Source: CAD feature listing. Evaluate the final solid. Frame: model axes, mm. A direction names the side the tool comes from. Round coordinates to 2 decimals unless told otherwise and drop trailing zeros. Order: outer loops, then holes, each group sorted by start corner. A loop starts at its lowest first (then second) coordinate and runs counter-clockwise, first axis right, second up. Notation, with made-up numbers: (-32, 0.25) -> (9, 0.25) arc R23 ccw to (9, 31.25) -> close; hole circle Ø3 at (-37.5, 51.25). An arc over 180 degrees is marked (long way). Answer as CSV lines item,"result". Start each with the question number.
(1) Contact query for flat-ended pins moving along their axis: P1, Ø6, axis at x = 6, z = -6, coming from the -Y side; P2, Ø2, axis at y = 19, z = 3, coming from the +X side; P3, Ø4, axis at y = 122, z = -4.5, coming from the +X side; P4, Ø8, axis at x = 8, z = -4, coming from the +Y side. Output: stop coordinate, or through.
(2) Section query A-A (y = 113). Output: boundary loops of the cut face in (x, z), plus the area to 3 significant figures.
(3) Pull-direction query (Y, two-part tool) for faces 5 (the flat face through (3, 119, 3)), 6 (the flat face through (9.93, 92.26, 0)), 7 (the cylindrical face through (-2.17, 124.39, 9.76)); classes: +Y half, -Y half, draft (parallel to the pull), parting line (faces both ways), or undercut.
(4) Line query: line 1 along Y through (x, z) = (-2, 4); line 2 along Y through (x, z) = (11, -1.5); line 3 along X through (y, z) = (82.5, -1.25). Output: solid intervals per line, ascending. Write a range as from..to.
(5) Set-up query: faces 1 (the flat face through (4, 122, 0.2)), 2 (the flat face through (2, 123.9, 2)), 3 (the flat face through (-0.2, 122, -4)), 4 (the flat face through (-0.003, 95.715, -9.877)). Return all of +Z, -Z, +X, -X, +Y, -Y with unobstructed straight access to the full face (end or side cutting, diameter ignored); none if empty.
```python
from build123d import *

# Parameters (mm, degrees)
EXTRUDE_START         = -0.2
EXTRUDE_1_OUTLINE_W   = 0.4
EXTRUDE_1_OUTLINE_H   = 3.7
EXTRUDE_1_DEPTH       = 0.4
EXTRUDE_START_2       = -7.2
EXTRUDE_1_2_OUTLINE_W = 0.4
EXTRUDE_1_2_OUTLINE_H = 3.7
EXTRUDE_1_2_DEPTH     = 7
EXTRUDE_START_3       = 119
EXTRUDE_1_3_OUTLINE_R = 14.4
EXTRUDE_1_3_DEPTH     = 1.2
EXTRUDE_1_4_OUTLINE_R = 14.5
EXTRUDE_1_4_DEPTH     = 0.85
EXTRUDE_START_4       = 123.9
EXTRUDE_1_5_OUTLINE_R = 10
EXTRUDE_1_5_DEPTH     = 1
EXTRUDE_1_6_DEPTH     = 0.4
CUT_EXTRUDE_1_DEPTH   = 129.075368436
CUT_EXTRUDE_2_DEPTH   = 129.075368436
DRAFT_1_ANGLE         = 63.434948823
DRAFT_2_ANGLE         = 63.434948823
RIB_1_REACH           = 130.053
SKETCH_4_WALL_W       = 267.026519706
SKETCH_4_WALL_H       = 0.4
RIB_2_REACH           = 130.053
SKETCH_5_WALL_W       = 267.026519706
SKETCH_5_WALL_H       = 0.4
RIB_3_REACH           = 130.053
SKETCH_6_WALL_W       = 267.026519706
SKETCH_6_WALL_H       = 0.4
RIB_4_REACH           = 130.053
SKETCH_7_WALL_W       = 261.805134662
SKETCH_7_WALL_H       = 0.4
RIB_5_REACH           = 130.053
SKETCH_8_WALL_W       = 261.805134662
SKETCH_8_WALL_H       = 0.4
RIB_6_REACH           = 130.053
SKETCH_9_WALL_W       = 261.805134662
SKETCH_9_WALL_H       = 0.4
RIB_START             = -0.2
RIB_7_DEPTH           = 0.4
RIB_8_DEPTH           = 0.4
FILLET_1_R            = 0.4
FILLET_2_R            = 2
FILLET_3_R            = 15


with BuildPart() as part:
    # 凸台-拉伸1: read off the stored shape, not the designer's step
    # 凸台-拉伸1 outline → 凸台-拉伸1 (new body)
    with BuildSketch(Plane.XY.offset(EXTRUDE_START)):
        Polygon((0, 126.4), (-0.2, 126.366666667), (-0.2, 124.9), (9, 124.9), (0.2, 126.366666667), align=None)
        with BuildLine():
            Line((13, 31), (13, 119))
            Line((13, 119), (-13, 119))
            Line((-13, 119), (-13, 20))
            Line((-13, 20), (-7.5, 20))
            Line((-7.5, 20), (-7.5, 2.391335203))
            ThreePointArc((-7.5, 2.391335203), (-7.838080215, 1.515615965), (-8.5, 0.85))
            Line((-8.5, 0.85), (8.5, 0.85))
            ThreePointArc((8.5, 0.85), (7.838080215, 1.515615965), (7.5, 2.391335203))
            Line((7.5, 2.391335203), (7.5, 31))
            Line((7.5, 31), (13, 31))
        make_face()
        with Locations((0, 122.05)):
            Rectangle(EXTRUDE_1_OUTLINE_W, EXTRUDE_1_OUTLINE_H)
    extrude(amount=EXTRUDE_1_DEPTH)

    # Extrude 1 2 outline → Extrude 1 2 (add)
    with BuildSketch(Plane.XY.offset(EXTRUDE_START_2)):
        with Locations((0, 122.05)):
            Rectangle(EXTRUDE_1_2_OUTLINE_W, EXTRUDE_1_2_OUTLINE_H)
    extrude(amount=EXTRUDE_1_2_DEPTH)

    # Extrude 1 3 outline → Extrude 1 3 (add)
    with BuildSketch(Plane(origin=(0, 0, 0), x_dir=(1, 0, 0), z_dir=(0, 1, 0)).offset(EXTRUDE_START_3)):
        Circle(EXTRUDE_1_3_OUTLINE_R)
    extrude(amount=EXTRUDE_1_3_DEPTH)

    # Extrude 1 4 outline → Extrude 1 4 (add)
    with BuildSketch(Plane(origin=(0, 0, 0), x_dir=(1, 0, 0), z_dir=(0, 1, 0))):
        Circle(EXTRUDE_1_4_OUTLINE_R)
    extrude(amount=EXTRUDE_1_4_DEPTH)

    # Extrude 1 5 outline → Extrude 1 5 (add)
    with BuildSketch(Plane(origin=(0, 0, 0), x_dir=(1, 0, 0), z_dir=(0, 1, 0)).offset(EXTRUDE_START_4)):
        Circle(EXTRUDE_1_5_OUTLINE_R)
    extrude(amount=EXTRUDE_1_5_DEPTH)

    # Extrude 1 6 outline → Extrude 1 6 (add)
    with BuildSketch(Plane.YZ.offset(EXTRUDE_START)):
        Polygon((126.366666667, -0.2), (126.4, 0), (126.366666667, 0.2), align=None)
    extrude(amount=EXTRUDE_1_6_DEPTH)

    # 草图2 → 切除-拉伸1 (cut, through all)
    with BuildSketch(Plane(origin=(0, 0, -0.2), x_dir=(-1, 0, 0), z_dir=(0, 0, -1))):
        with BuildLine():
            Line((-13, 90.7), (-7.905050667, 93.286666585))
            ThreePointArc((-7.905050667, 93.286666585), (-7.467204555, 94), (-7.905050667, 94.713333415))
            Line((-7.905050667, 94.713333415), (-13, 97.3))
            Line((-13, 97.3), (-13, 90.7))
        make_face()
    extrude(amount=-CUT_EXTRUDE_1_DEPTH, mode=Mode.SUBTRACT)

    # 草图3 → 切除-拉伸2 (cut, through all)
    with BuildSketch(Plane(origin=(0, 0, -0.2), x_dir=(-1, 0, 0), z_dir=(0, 0, -1))):
        with BuildLine():
            Line((13, 97.3), (7.905050667, 94.713333415))
            ThreePointArc((7.905050667, 94.713333415), (7.467204555, 94), (7.905050667, 93.286666585))
            Line((7.905050667, 93.286666585), (13, 90.7))
            Line((13, 90.7), (13, 97.3))
        make_face()
    extrude(amount=-CUT_EXTRUDE_2_DEPTH, mode=Mode.SUBTRACT)

    # 拔模1
    draft_1_faces = [part.faces().sort_by_distance(p)[0] for p in [
        (-10.25, 20, 0),
    ]]
    draft(draft_1_faces, Plane(origin=(-7.5, 0, -0.2), x_dir=(0, 0, -1), z_dir=(-1, 0, 0)), DRAFT_1_ANGLE)

    # 拔模2
    draft_2_faces = [part.faces().sort_by_distance(p)[0] for p in [
        (10.25, 31, 0),
    ]]
    draft(draft_2_faces, Plane(origin=(13, 0, 0.2), x_dir=(0, 0, 1), z_dir=(1, 0, 0)), DRAFT_2_ANGLE)

    # 草图4 wall → 筋1 (add, up to next)
    with BuildSketch(Plane(origin=(0, 125.633333334, 4.6), x_dir=(0, -0.164398987342, 0.986393923826), z_dir=(0, -0.986393923826, -0.164398987342)), mode=Mode.PRIVATE) as rib_1_sk1:
        Rectangle(SKETCH_4_WALL_W, SKETCH_4_WALL_H)
    rib_1_tool1 = extrude(rib_1_sk1.sketch, amount=RIB_1_REACH, mode=Mode.PRIVATE) - part.part
    add(rib_1_tool1.solids().sort_by_distance((0, 125.633333334, 4.6))[0])

    # 草图5 wall → 筋2 (add, up to next)
    with BuildSketch(Plane(origin=(-4.6, 125.633333334, 0), x_dir=(0.986393923826, 0.164398987342, 0), z_dir=(0.164398987342, -0.986393923826, 0)), mode=Mode.PRIVATE) as rib_2_sk1:
        Rectangle(SKETCH_5_WALL_W, SKETCH_5_WALL_H)
    rib_2_tool1 = extrude(rib_2_sk1.sketch, amount=RIB_2_REACH, mode=Mode.PRIVATE) - part.part
    add(rib_2_tool1.solids().sort_by_distance((-4.6, 125.633333334, 0))[0])

    # 草图6 wall → 筋3 (add, up to next)
    with BuildSketch(Plane(origin=(0, 125.633333334, -4.6), x_dir=(0, 0.164398987342, 0.986393923826), z_dir=(0, -0.986393923826, 0.164398987342)), mode=Mode.PRIVATE) as rib_3_sk1:
        Rectangle(SKETCH_6_WALL_W, SKETCH_6_WALL_H)
    rib_3_tool1 = extrude(rib_3_sk1.sketch, amount=RIB_3_REACH, mode=Mode.PRIVATE) - part.part
    add(rib_3_tool1.solids().sort_by_distance((0, 125.633333334, -4.6))[0])

    # 草图7 wall → 筋4 (add, up to next)
    with BuildSketch(Plane(origin=(-7.2, 122.05, 0), x_dir=(0, -1, 0), z_dir=(1, 0, 0)), mode=Mode.PRIVATE) as rib_4_sk1:
        Rectangle(SKETCH_7_WALL_W, SKETCH_7_WALL_H)
    rib_4_tool1 = extrude(rib_4_sk1.sketch, amount=RIB_4_REACH, mode=Mode.PRIVATE) - part.part
    add(rib_4_tool1.solids().sort_by_distance((-7.2, 122.05, 0))[0])

    # 草图8 wall → 筋5 (add, up to next)
    with BuildSketch(Plane(origin=(0, 122.05, 7.2), x_dir=(0, -1, 0), z_dir=(0, 0, -1)), mode=Mode.PRIVATE) as rib_5_sk1:
        Rectangle(SKETCH_8_WALL_W, SKETCH_8_WALL_H)
    rib_5_tool1 = extrude(rib_5_sk1.sketch, amount=RIB_5_REACH, mode=Mode.PRIVATE) - part.part
    add(rib_5_tool1.solids().sort_by_distance((0, 122.05, 7.2))[0])

    # 草图9 wall → 筋6 (add, up to next)
    with BuildSketch(Plane(origin=(7.2, 122.05, 0), x_dir=(0, -1, 0), z_dir=(-1, 0, 0)), mode=Mode.PRIVATE) as rib_6_sk1:
        Rectangle(SKETCH_9_WALL_W, SKETCH_9_WALL_H)
    rib_6_tool1 = extrude(rib_6_sk1.sketch, amount=RIB_6_REACH, mode=Mode.PRIVATE) - part.part
    add(rib_6_tool1.solids().sort_by_distance((7.2, 122.05, 0))[0])

    # 筋7: read off the stored shape, not the designer's step
    # 筋7 outline → 筋7 (add)
    with BuildSketch(Plane(origin=(0, 0, 0), x_dir=(0, 0, -1), z_dir=(1, 0, 0)).offset(RIB_START)):
        with BuildLine():
            Line((7.905050667, 94.713333415), (13, 97.3))
            Line((13, 97.3), (13, 119))
            Line((13, 119), (0.2, 119))
            Line((0.2, 119), (0.2, 0.85))
            Line((0.2, 0.85), (8.5, 0.85))
            ThreePointArc((8.5, 0.85), (7.838080215, 1.515615965), (7.5, 2.391335203))
            Line((7.5, 2.391335203), (7.5, 20))
            Line((7.5, 20), (13, 31))
            Line((13, 31), (13, 90.7))
            Line((13, 90.7), (7.905050667, 93.286666585))
            ThreePointArc((7.905050667, 93.286666585), (7.467204555, 94), (7.905050667, 94.713333415))
        make_face()
    extrude(amount=RIB_7_DEPTH)

    # 筋8: read off the stored shape, not the designer's step
    # 筋8 outline → 筋8 (add)
    with BuildSketch(Plane(origin=(0, 0, 0), x_dir=(0, -1, 0), z_dir=(-1, 0, 0)).offset(RIB_START)):
        with BuildLine():
            Line((-94.713333415, 7.905050667), (-97.3, 13))
            Line((-97.3, 13), (-119, 13))
            Line((-119, 13), (-119, 0.2))
            Line((-119, 0.2), (-0.85, 0.2))
            Line((-0.85, 0.2), (-0.85, 8.5))
            ThreePointArc((-0.85, 8.5), (-1.515615965, 7.838080215), (-2.391335203, 7.5))
            Line((-2.391335203, 7.5), (-20, 7.5))
            Line((-20, 7.5), (-31, 13))
            Line((-31, 13), (-90.7, 13))
            Line((-90.7, 13), (-93.286666585, 7.905050667))
            ThreePointArc((-93.286666585, 7.905050667), (-94, 7.467204555), (-94.713333415, 7.905050667))
        make_face()
    extrude(amount=RIB_8_DEPTH)

    # 圆角1
    fillet_1_edges = [part.edges().sort_by_distance(p)[0] for p in [
        (-14.5, 0, 0),
        (-14.5, 0.85, 0),
    ]]
    fillet(fillet_1_edges, radius=FILLET_1_R)

    # 圆角2
    fillet_2_edges = [part.edges().sort_by_distance(p)[0] for p in [
        (13, 90.7, 0),
        (13, 97.3, 0),
        (-13, 97.3, 0),
        (-13, 90.7, 0),
        (0, 90.7, -13),
        (0, 97.3, -13),
        (0, 90.7, 13),
        (0, 97.3, 13),
    ]]
    fillet(fillet_2_edges, radius=FILLET_2_R)

    # 圆角3
    fillet_3_edges = [part.edges().sort_by_distance(p)[0] for p in [
        (-13, 31, 0),
        (-7.5, 20, 0),
        (7.5, 20, 0),
        (13, 31, 0),
        (0, 20, -7.5),
        (0, 31, -13),
        (0, 20, 7.5),
        (0, 31, 13),
    ]]
    fillet(fillet_3_edges, radius=FILLET_3_R)


solid = part.part
```
Answer block:
1,P1,"y = 0"
1,P2,"x = 0.2"
1,P3,"x = 13.94"
1,P4,"y = 125.27"
2,outline,"(-13, -0.2) -> (-0.2, -0.2) -> (-0.2, -13) -> (0.2, -13) -> (0.2, -0.2) -> (13, -0.2) -> (13, 0.2) -> (0.2, 0.2) -> (0.2, 13) -> (-0.2, 13) -> (-0.2, 0.2) -> (-13, 0.2) -> close"
2,area,"20.6 mm2"
3,face 5,"undercut"
3,face 6,"undercut"
3,face 7,"draft"
4,line 1,"0..0.85, 119..120.2, 123.9..124.9"
4,line 2,"0..0.85, 119..120.2"
4,line 3,"-0.2..0.2"
5,face 1,"+Z, +X"
5,face 2,"none"
5,face 3,"-Z, -X"
5,face 4,"-Z, +X, -X"
